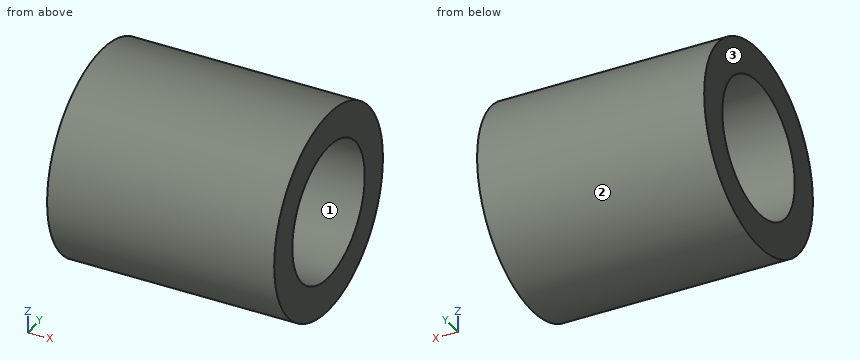
Autodesk Fusion 360 part; units mm, degrees
sketch "Sketch1" plane through (0, 0, 0) normal (1, 0, 0) x (0, 0, -1)
  circle A0 centre (0, 0) radius 6
  circle A1 centre (0, 0) radius 9
  dimension "d1" = 12
  dimension "d2" = 18
extrude "Extrude1" add sketch "Sketch1" along normal blind 20 makes body 1
copy_body "Body->Comp1" bodies 1 removing the originals makes body 2 in component "12x18x20 bushing"
component "12x18x20 bushing" placed x (1, 0, 0) y (0, 1, 0) z (0, 0, 1) at (0, 0, 0)
Input: part model. Units: mm. Frame: model coordinates. Face numbers are marked on the shaded views. Coordinates: 2 decimals unless noted, no trailing zeros. Write each loop counter-clockwise with the first axis right and the second up, starting at its lowest first coordinate (ties: lowest second). Pieces come first, ordered by that corner, then holes.
1) Section C-C on x = 8.25. Output: boundary loops of the cut face in (y, z).
2) Mould query, pull axis Y, two halves, no side actions, for the marked faces 1, 2 and 3. Classes: pulls with the +Y half, pulls with the -Y half, needs draft (parallel to the pull), parting line crosses it, or undercut.
3) Section D-D on y = -6.5. Output: boundary loops of the cut face in (x, z).
4) Section A-A on y = 0. Output: boundary loops of the cut face in (x, z).
5) Material intervals for line 1 along Y through (x, z) = (6.25, 0); line 2 along Z through (x, y) = (2, -0.25); line 3 along Y through (x, z) = (7.75, 2.5), sorted ascending.
6) Pin query (flat end, axial travel): pin 1 Ø4 at (x, y) = (17.5, 3.5) entering from +Z; pin 2 Ø1 at (x, z) = (4.5, -2.5) entering from -Y; pin 3 Ø1 at (x, z) = (11.5, -2.5) entering from +Y; pin 4 Ø6 at (x, y) = (13.5, 2.5) entering from -Z. Return the tip coordinate at first contact, or that it passes through.
Check result:
1. outline: circle Ø18 at (0, 0); hole circle Ø12 at (0, 0)
2. face 1: undercut
2. face 2: parting line crosses it
2. face 3: needs draft
3. outline: (0, -6.22) - (20, -6.22) - (20, 6.22) - (0, 6.22) - close
4. outline: (0, -9) - (20, -9) - (20, -6) - (0, -6) - close; (0, 6) - (20, 6) - (20, 9) - (0, 9) - close
5. line 1: y = -9 to -6, 6 to 9
5. line 2: z = -9 to -5.99, 5.99 to 9
5. line 3: y = -8.65 to -5.45, 5.45 to 8.65
6. pin 1: stops at z = 8.87
6. pin 2: stops at y = -8.77
6. pin 3: stops at y = 8.77
6. pin 4: stops at z = -9
